Geometry check sheet. Reference: the model listing, model coordinates, mm. A direction names the side the tool comes from. Round coordinates to 2 decimals unless told otherwise and drop trailing zeros. Write each loop counter-clockwise with the first axis right and the second up, starting at its lowest first coordinate (ties: lowest second). Pieces come first, ordered by that corner, then holes. Notation, with made-up numbers: (20.5, -29) -> (37.5, -29) arc R19 ccw to (37.5, 7) -> close; hole circle Ø8 at (46, 4). An arc over 180 degrees is marked (long way). Use a Markdown table: item, result.
```python
from build123d import *

# Parameters (mm, degrees)
F0_W     = 25.4
F0_H     = 38.1
F1_DEPTH = 12.7
F2_R     = 3.301742
F3_DEPTH = 25.4
F4_R     = 2.696389
F5_DEPTH = 25.4


with BuildPart() as f1:
    # F0 (on Front) → F1 (new body)
    with BuildSketch(Plane.XZ):
        with Locations((3.099383, 0.865355)):
            Rectangle(F0_W, F0_H)
    extrude(amount=F1_DEPTH)

    # F2 (on face) → F3 (cut)
    with BuildSketch(Plane.XZ.offset(12.7)):
        with Locations((3.099383, -5.484645)):
            Circle(F2_R)
    extrude(amount=-F3_DEPTH, mode=Mode.SUBTRACT)

    # F4 (on face) → F5 (cut)
    with BuildSketch(Plane.XY.offset(19.915355)):
        with Locations((3.099383, -6.35)):
            Circle(F4_R)
    extrude(amount=-F5_DEPTH, mode=Mode.SUBTRACT)


solid = f1.part
```
(1) Gauge pin test, flat end, axial feed: pin 1 Ø3 at (x, y) = (3.1, -6.35) entering from +Z. Record the tip position at first contact, or that the pin passes through.
A:
| item | result |
|---|---|
| pin 1 | stops at z = -8.43 |
(2) Section check A-A on z = 0.5. Record the cut outline in (x, y).
A:
| item | result |
|---|---|
| outline | (-9.6, -12.7) -> (15.8, -12.7) -> (15.8, 0) -> (-9.6, 0) -> close; hole circle Ø5.39 at (3.1, -6.35) |
(3) Section check B-B on y = -6.35. Record the cut outline in (x, z), plus the area to 3 significant figures.
A:
| item | result |
|---|---|
| outline | (-9.6, -18.18) -> (15.8, -18.18) -> (15.8, 19.92) -> (5.8, 19.92) -> (5.8, -3.58) arc R3.3 cw (long way) to (0.4, -3.58) -> (0.4, 19.92) -> (-9.6, 19.92) -> close |
| area | 812 mm2 |
(4) Release check for a two-part mould opening along Z. For faces 3 (the face through (0, -6, 19.915)), 4 (the face through (2.384, -6.439, -8.708)), 5 (the face through (15.799, -6, 1)) record: +Z half, -Z half, draft (parallel to the pull), parting line (faces both ways), or undercut.
A:
| item | result |
|---|---|
| face 3 | +Z half |
| face 4 | undercut |
| face 5 | draft |
(5) Access from +Z, -Z, +X, -X, +Y, -Y to the whole of each face (thin tool, end or side, straight path). Record for faces 1 (the face through (2.748, -3.677, 8.333)), 2 (the face through (3, -12.7, 1)).
A:
| item | result |
|---|---|
| face 1 | +Z |
| face 2 | +Z, -Z, +X, -X, -Y |
(6) Section check C-C on y = -2.75. Record the cut outline in (x, z).
A:
| item | result |
|---|---|
| outline | (-9.6, -18.18) -> (15.8, -18.18) -> (15.8, 19.92) -> (-9.6, 19.92) -> close; hole circle Ø6.6 at (3.1, -5.48) |
(7) Thickness scan on line 1 (X direction, y = -2, z = -5.5); line 2 (X direction, y = -6.35, z = 11.25); line 3 (Y direction, x = 3.5, z = 16). Record the ranges inside material, lowest first.
A:
| item | result |
|---|---|
| line 1 | x = -9.6 to -0.2, 6.4 to 15.8 |
| line 2 | x = -9.6 to 0.4, 5.8 to 15.8 |
| line 3 | y = -12.7 to -9.02, -3.68 to 0 |
